Work out the finished part from the listing and answer in its coordinate system (mm). Face numbers are marked on the shaded views. A direction names the side the tool comes from. Round coordinates to 2 decimals unless told otherwise and drop trailing zeros. Order: outer loops, then holes, each group sorted by start corner. A loop starts at its lowest first (then second) coordinate and runs counter-clockwise, first axis right, second up. Notation, with made-up numbers: (43, 0) - (96, 0) arc R35 cw to (96, 33) - close; hole circle Ø6 at (-32.75, 71). An arc over 180 degrees is marked (long way). Answer in a Markdown table with one row per item.
from build123d import *

# Parameters (mm, degrees)
ESQUISSE1_W                                    = 25
ESQUISSE1_H                                    = 8
BOSS_EXTRU_1_DEPTH                             = 12
FRAISAGE_POUR_VIS_T_TE_FRAIS_E_M31_D           = 3.4
FRAISAGE_POUR_VIS_T_TE_FRAIS_E_M31_CSINK_D     = 6.3
FRAISAGE_POUR_VIS_T_TE_FRAIS_E_M31_CSINK_ANGLE = 90
ENL_V_MAT_EXTRU_1_DEPTH                        = 13
CHANFREIN1_SIZE                                = 1


with BuildPart() as part:
    # Esquisse1 → Boss.-Extru.1 (new body)
    with BuildSketch(Plane.XY):
        Rectangle(ESQUISSE1_W, ESQUISSE1_H)
    extrude(amount=BOSS_EXTRU_1_DEPTH)

    # Fraisage pour vis à tête fraisée M31 (through all)
    with Locations(Plane(origin=(0, 4, 0), x_dir=(1, 0, 0), z_dir=(0, 1, 0))):
        with Locations((0, -6)):
            CounterSinkHole(FRAISAGE_POUR_VIS_T_TE_FRAIS_E_M31_D / 2, FRAISAGE_POUR_VIS_T_TE_FRAIS_E_M31_CSINK_D / 2, counter_sink_angle=FRAISAGE_POUR_VIS_T_TE_FRAIS_E_M31_CSINK_ANGLE)

    # Esquisse4 → Enlèv. mat.-Extru.1 (cut, through all)
    with BuildSketch(Plane.XY.offset(12)):
        with BuildLine():
            Line((-5.25, -1), (-5.25, -4))
            Line((-5.25, -4), (-10.75, -4))
            Line((-10.75, -4), (-10.75, -1))
            ThreePointArc((-10.75, -1), (-8, 1.75), (-5.25, -1))
        make_face()
        with BuildLine():
            Line((5.25, -1), (5.25, -4))
            Line((5.25, -4), (10.75, -4))
            Line((10.75, -4), (10.75, -1))
            ThreePointArc((10.75, -1), (8, 1.75), (5.25, -1))
        make_face()
    extrude(amount=-ENL_V_MAT_EXTRU_1_DEPTH, mode=Mode.SUBTRACT)

    # Chanfrein1
    chanfrein1_edges = [part.edges().sort_by_distance(p)[0] for p in [
        (-12.5, 0, 12),
        (12.5, 0, 12),
        (-12.5, 0, 0),
        (0, 4, 0),
        (12.5, 0, 0),
        (-12.5, 4, 6),
        (12.5, 4, 6),
        (0, 4, 12),
    ]]
    chamfer(chanfrein1_edges, length=CHANFREIN1_SIZE)


solid = part.part
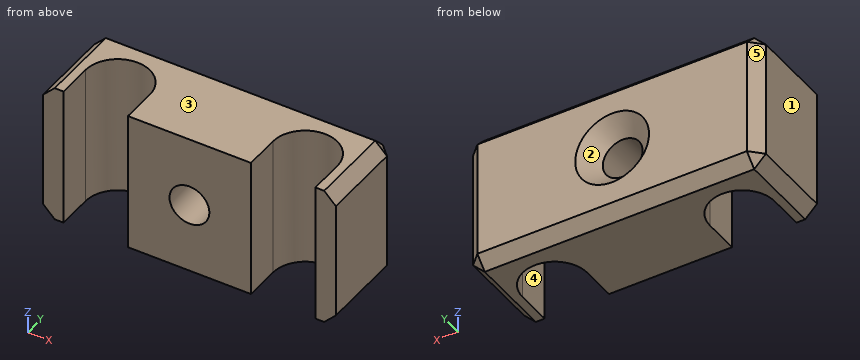
1) Find section D-D, the plane y = 3.5. Give the vertices of the cut face in (x, z).
Filled in:
| item | result |
|---|---|
| outline | (-12, 1) - (-11.5, 0.5) - (11.5, 0.5) - (12, 1) - (12, 11) - (11.5, 11.5) - (-11.5, 11.5) - (-12, 11) - close; hole circle Ø5.3 at (0, 6) |
2) The mould has two halves that part along X. Classify the marked faces 1, 2 and 3: released by +X, released by -X, zero draft, split by the parting line, or undercut.
Filled in:
| item | result |
|---|---|
| face 1 | released by -X |
| face 2 | undercut |
| face 3 | zero draft |
3) Each of these flat-tipped pins is pushed along its axis until it touches: pin 1 (1.5 mm diameter, centred on x = -3, y = -2, fed in from -Z); pin 2 (4 mm diameter, centred on x = -8, z = 7.5, fed in from -Y); pin 3 (3 mm diameter, centred on x = 9, z = 3, fed in from -Y). Where does it stop, or does it pass through?
Filled in:
| item | result |
|---|---|
| pin 1 | stops at z = 0 |
| pin 2 | stops at y = 0.89 |
| pin 3 | stops at y = 0.15 |
4) Find section C-C, the plane x = 0. Give the vertices of the cut face in (y, z), then the cut area to 3 significant figures.
Filled in:
| item | result |
|---|---|
| outline | (-4, 0) - (3, 0) - (4, 1) - (4, 2.85) - (2.55, 4.3) - (-4, 4.3) - close; (-4, 7.7) - (2.55, 7.7) - (4, 9.15) - (4, 11) - (3, 12) - (-4, 12) - close |
| area | 65.7 mm^2 |
5) Find the intervals of material crossed by probe 1 along X at (y, z) = (-2, 6); probe 2 along X at (y, z) = (-1, 10.5), in increasing order. Write a range as from..to.
Filled in:
| item | result |
|---|---|
| probe 1 | x = -12.5..-10.75, -5.25..-1.7, 1.7..5.25, 10.75..12.5 |
| probe 2 | x = -12.5..-10.75, -5.25..5.25, 10.75..12.5 |
6) Which of the six approach directions +Z, -Z, +X, -X, +Y, -Y give full straight-line access (tool end or side, diameter ignored) to the marked faces 4 and 5?
Filled in:
| item | result |
|---|---|
| face 4 | +Z, -Z, -Y |
| face 5 | +Z, -Z, -X, +Y |
7) Find section A-A, the plane y = -2.5. Give the vertices of the cut face in (x, z), then the cut area to 3 significant figures.
Filled in:
| item | result |
|---|---|
| outline | (-12.5, 1) - (-11.5, 0) - (-10.75, 0) - (-10.75, 12) - (-11.5, 12) - (-12.5, 11) - close; (-5.25, 0) - (5.25, 0) - (5.25, 12) - (-5.25, 12) - close; (10.75, 0) - (11.5, 0) - (12.5, 1) - (12.5, 11) - (11.5, 12) - (10.75, 12) - close; hole circle Ø3.4 at (0, 6) |
| area | 157 mm^2 |
8) Find section B-B, the plane z = 6. Give the vertices of the cut face in (x, y), then the cut area to 3 significant figures.
Filled in:
| item | result |
|---|---|
| outline | (-12.5, -4) - (-10.75, -4) - (-10.75, -1) arc R2.75 cw to (-5.25, -1) - (-5.25, -4) - (-1.7, -4) - (-1.7, 2.55) - (-3.15, 4) - (-11.5, 4) - (-12.5, 3) - close; (1.7, -4) - (5.25, -4) - (5.25, -1) arc R2.75 cw to (10.75, -1) - (10.75, -4) - (12.5, -4) - (12.5, 3) - (11.5, 4) - (3.15, 4) - (1.7, 2.55) - close |
| area | 113 mm^2 |
